The model under review builds one solid part; all positions refer to its coordinate system, in mm. Face numbers are marked on the shaded views. A direction names the side the tool comes from. Round coordinates to 2 decimals unless told otherwise and drop trailing zeros. Loops run counter-clockwise (first coordinate to the right, second up) from the corner with the lowest first, then second, coordinate; pieces in that order, holes last. Notation, with made-up numbers: M 0.25,81.25 L 23.25,81.25 A13 cw 23.25,104.25 Z; hole C -16.75,-12.75 d11. An arc over 180 degrees is marked long. Answer as a JSON object with one key per item and string values. Group by question number.
Item 1: Consider section D-D (x = 10). Give the boundary of the cut face in (y, z).
Item 2: To check wall thickness, follow line 1 (Y direction, x = 6.5, z = 42.5); line 2 (Y direction, x = 40, z = 70.5); line 3 (X direction, y = -24, z = 24). State the ranges of each line that lie inside material, in increasing order.
Item 3: Consider section A-A (x = 36). Give the boundary of the cut face in (y, z).
Item 4: Consider section C-C (z = 58). Give the boundary of the cut face in (x, y), and give its area (3 significant figures).
Item 5: Tool access review of the marked faces 1, 2, 3 and 4: name each direction out of +Z, -Z, +X, -X, +Y, -Y from which nothing blocks a thin tool from reaching the whole face with its end or side.
Item 6: Insertion check: P1, Ø12, axis at x = 67.5, z = 74.5, coming from the +Y side; P2, Ø12, axis at x = 33, y = -13, coming from the +Z side; P3, Ø18, axis at x = 30, z = 39.5, coming from the -Y side; P4, Ø2, axis at y = -45, z = 50.5, coming from the +X side. Each pin has a flat end and moves straight along its axis. Give the tip position at first contact, or say it passes through.
Item 7: Consider section B-B (y = -55.5). Give the boundary of the cut face in (x, z), and give its area (3 significant figures).
```python
from build123d import *

# Parameters (mm, degrees)
F0_W     = 60
F0_H     = 60
F1_DEPTH = 60
F2_W     = 30
F2_H     = 30


with BuildPart() as f1:
    # F0 (on Front) → F1 (new body)
    with BuildSketch(Plane.XZ):
        with Locations((30, 30)):
            Rectangle(F0_W, F0_H)
    extrude(amount=F1_DEPTH)

    # F2 (on face) → F3 (revolve)
    with BuildSketch(Plane.XY.offset(60)):
        with Locations((75, -52.221692)):
            Rectangle(F2_W, F2_H)
    revolve(axis=Axis((60, -52.221692, 60), (0, -1, 0)))


solid = f1.part
```
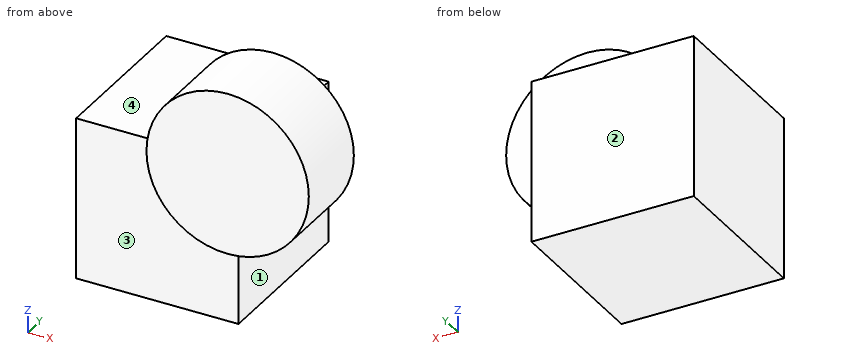
Geometry results:
{
 "1": {"outline": "M -60,0 L 0,0 L 0,60 L -60,60 Z"},
 "2": {"line 1": "y = -60 to 0", "line 2": "y = -67.22 to -37.22", "line 3": "x = 0 to 60"},
 "3": {"outline": "M -67.22,42 L -60,42 L -60,0 L 0,0 L 0,60 L -37.22,60 L -37.22,78 L -67.22,78 Z"},
 "4": {"outline": "M 0,-60 L 30.07,-60 L 30.07,-67.22 L 89.93,-67.22 L 89.93,-37.22 L 60,-37.22 L 60,0 L 0,0 Z", "area": "4,710 mm^2"},
 "5": {"face 1": "-Z, +X, +Y", "face 2": "+Z, -Z, +X, -X, +Y", "face 3": "-Z, -X, -Y", "face 4": "+Z, -X, +Y"},
 "6": {"P1": "stops at y = -37.22", "P2": "stops at z = 60", "P3": "stops at y = -67.22", "P4": "stops at x = 88.77"},
 "7": {"outline": "M 0,0 L 60,0 L 60,30 A30 ccw long 30,60 L 0,60 Z", "area": "5,720 mm^2"}
}
